Build history of the part. All positions in model axes, mm. Round coordinates to 2 decimals unless told otherwise and drop trailing zeros. Loops run counter-clockwise (first coordinate to the right, second up) from the corner with the lowest first, then second, coordinate; pieces in that order, holes last. Notation, with made-up numbers: (0.5, 16.25) -> (53.5, 16.25) arc R26 ccw to (53.5, 48.25) -> close; hole circle Ø1 at (0, 68). An arc over 180 degrees is marked (long way). Put each result on its own line as item: value. Start each with the question number.
Item 1: Flat gauge pins, fed straight in: pin 1 Ø12 at (x, z) = (-4.5, 379.5) entering from +Y; pin 2 Ø8 at (y, z) = (-19.5, 93) entering from +X; pin 3 Ø7.5 at (x, z) = (12, 718) entering from +Y (3 decimals). Where does each tip first touch, or does it go through?
Item 2: Cut at D-D, the plane y = -20. List the corners of the cut face in (x, z) (3 decimals).
Item 3: Cut at A-A, the plane x = 13. List the corners of the cut face in (y, z) (3 decimals).
Item 4: Cut at B-B, the plane y = 9.5. List the corners of the cut face in (x, z) (3 decimals), plus the area to 3 significant figures.
Item 5: Cut at C-C, the plane z = 492. List the corners of the cut face in (x, y) (3 decimals).
Item 6: Drill centre lines: probe 1 along X at (y, z) = (-24, 235) (3 decimals); probe 2 along Y at (x, z) = (-15.5, 427) (3 decimals); probe 3 along X at (y, z) = (2, 158) (3 decimals). Where is each one in solid material? Low to high. Write a range as [from, to].
Autodesk Fusion 360 part; units mm, degrees
sketch "Sketch2" plane through (0, 0, 0) normal (0, 0, 1) x (1, 0, 0)
  line L0 (-34.925, 34.925) -> (34.925, 34.925)
  line L1 (34.925, 34.925) -> (34.925, -34.925)
  line L2 (34.925, -34.925) -> (-34.925, -34.925)
  line L3 (-34.925, -34.925) -> (-34.925, 34.925)
  line L4 (-34.925, 34.925) -> (34.925, -34.925) construction
  line L5 (34.925, 34.925) -> (-34.925, -34.925) construction
  dimension "d1" = 69.85
  dimension "d2" = 69.85
extrude "Extrude1" add sketch "Sketch2" along normal blind 762
chamfer "Chamfer1" distance 31.75 distance2 609.6 2 edges at (34.925, 0, 0) (0, 34.925, 0) measured on face at (11.6417, -11.6417, 0) measured on face at (11.6417, -11.6417, 0)
sketch "Sketch6" plane through (34.925, 0, 0) normal (1, 0, 0) x (0, 1, 0)
  line L0 (-34.925, 609.6) -> (34.925, 609.6)
  line L1 (34.925, 609.6) -> (34.925, 762)
  line L2 (34.925, 762) -> (-34.925, 762)
  line L3 (-34.925, 762) -> (-34.925, 609.6)
  line L4 (-34.925, 762) -> (-34.925, 723.9) construction
  line L5 (-34.925, 723.9) -> (12.7, 723.9) construction
  line L6 (3.175, 736.6) -> (22.225, 736.6)
  line L7 (22.225, 736.6) -> (22.225, 711.2)
  line L8 (22.225, 711.2) -> (3.175, 711.2)
  line L9 (3.175, 711.2) -> (3.175, 736.6)
  line L10 (3.175, 736.6) -> (22.225, 711.2) construction
  line L11 (22.225, 736.6) -> (3.175, 711.2) construction
  point P0 (12.7, 723.9)
  dimension "d23" = 38.1
  dimension "d24" = 47.625
  dimension "d25" = 19.05
  dimension "d26" = 25.4
extrude "Extrude5" cut sketch "Sketch6" against normal blind 31.75 contours L6 L7 L8 L9
sketch "Sketch7" plane through (0, 34.925, 0) normal (0, 1, 0) x (-1, 0, 0)
  line L0 (-34.925, 609.6) -> (34.925, 609.6)
  line L1 (34.925, 609.6) -> (34.925, 762)
  line L2 (34.925, 762) -> (-34.925, 762)
  line L3 (-34.925, 762) -> (-34.925, 609.6)
  line L4 (34.925, 762) -> (34.925, 723.9) construction
  line L5 (34.925, 723.9) -> (-12.7, 723.9) construction
  line L6 (-22.225, 736.6) -> (-3.175, 736.6)
  line L7 (-3.175, 736.6) -> (-3.175, 711.2)
  line L8 (-3.175, 711.2) -> (-22.225, 711.2)
  line L9 (-22.225, 711.2) -> (-22.225, 736.6)
  line L10 (-22.225, 736.6) -> (-3.175, 711.2) construction
  line L11 (-3.175, 736.6) -> (-22.225, 711.2) construction
  point P0 (-12.7, 723.9)
  dimension "d29" = 38.1
  dimension "d30" = 47.625
  dimension "d31" = 19.05
  dimension "d32" = 25.4
extrude "Extrude6" cut sketch "Sketch7" against normal blind 31.75 contours L6 L7 L8 L9
equation "d24 = 1.125 in + 0.375 in + 0.375 in"
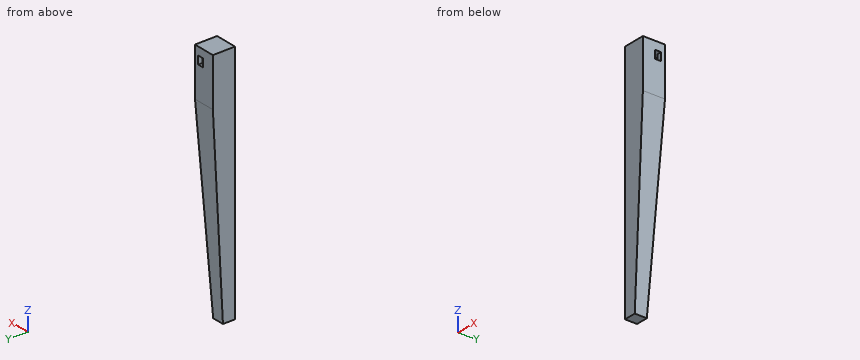
Reply:
1. pin 1: stops at y = 23.25
1. pin 2: stops at x = 8.23
1. pin 3: stops at y = 3.175
2. outline: (-34.925, 0) -> (3.175, 0) -> (34.925, 609.6) -> (34.925, 762) -> (-34.925, 762) -> close
3. outline: (-34.925, 188.64) -> (13, 188.64) -> (34.925, 609.6) -> (34.925, 711.2) -> (3.175, 711.2) -> (3.175, 736.6) -> (34.925, 736.6) -> (34.925, 762) -> (-34.925, 762) -> close
4. outline: (-34.925, 121.44) -> (9.5, 121.44) -> (34.925, 609.6) -> (34.925, 711.2) -> (3.175, 711.2) -> (3.175, 736.6) -> (34.925, 736.6) -> (34.925, 762) -> (-34.925, 762) -> close
4. area: 37,700 mm^2
5. outline: (-34.925, -34.925) -> (28.8, -34.925) -> (28.8, 28.8) -> (-34.925, 28.8) -> close
6. probe 1: x = [-34.925, 15.415]
6. probe 2: y = [-34.925, 25.415]
6. probe 3: x = [-34.925, 11.404]
